Part model, mm, in its own coordinate system. Face numbers are marked on the shaded views. Round coordinates to 2 decimals unless told otherwise and drop trailing zeros. Order: outer loops, then holes, each group sorted by start corner. A loop starts at its lowest first (then second) coordinate and runs counter-clockwise, first axis right, second up. Notation, with made-up numbers: (7, 43) - (23, 43) arc R15 ccw to (23, 71) - close; hole circle Ø7 at (57.5, 6). An arc over 180 degrees is marked (long way). Answer as a JSON object with one key per item and string values.
Autodesk Inventor part; units mm, degrees
ref_plane "Start Plane" through (0, 0, -10) normal (0, 0, 1) x (1, 0, 0)
ref_plane "End Plane" through (0, 0, 140) normal (0, 0, 1) x (1, 0, 0)
ref_plane "Work Plane4" through (0, 0, -10) normal (0, 0, -1) x (-1, 0, 0)
ref_plane "Start Plane" through (0, 0, -10) normal (0, 0, 1) x (1, 0, 0)
ref_plane "End Plane" through (0, 0, 140) normal (0, 0, 1) x (1, 0, 0)
sketch "Sketch" plane through (0, 0, 0) normal (0, 0, 1) x (1, 0, 0)
  line L0 (-10, -7) -> (-10, 7)
  line L1 (-7, 10) -> (7, 10)
  line L2 (10, 7) -> (10, -7)
  line L3 (7, -10) -> (-7, -10)
  arc A0 (-10, -7) -> (-7, -10) centre (-7, -7) ccw
  arc A1 (-7, 10) -> (-10, 7) centre (-7, 7) ccw
  arc A2 (10, 7) -> (7, 10) centre (7, 7) ccw
  arc A3 (7, -10) -> (10, -7) centre (7, -7) ccw
  arc A4 (-7, 8) -> (-8, 7) centre (-7, 7) ccw
  line L4 (-7, 8) -> (7, 8)
  arc A5 (8, 7) -> (7, 8) centre (7, 7) ccw
  line L5 (8, 7) -> (8, -7)
  arc A6 (7, -8) -> (8, -7) centre (7, -7) ccw
  line L6 (7, -8) -> (-7, -8)
  arc A7 (-8, -7) -> (-7, -8) centre (-7, -7) ccw
  line L7 (-8, -7) -> (-8, 7)
  line L8 (0, 14.8698) -> (0, -14.8698) construction
  line L9 (-14.8698, 0) -> (14.8698, 0) construction
  dimension "d7" = 3
  dimension "d10" = 20
  dimension "d11" = 20
  dimension "d12" = 2
  dimension "d15" = 10
  dimension "d16" = 10
extrude "Body" add sketch "Sketch" along normal up to surface (150 mm away) from surface at -10
sketch "Sketch3" plane through (0, 0, 0) normal (0, 0, 1) x (1, 0, 0)
  line L0 (0, 0) -> (10, 0)
ref_plane "Work Plane3" through (0, 0, 0) normal (0, -1, 0) x (1, 0, 0)
sketch "Sketch4" plane through (0, 0, 0) normal (0, -1, 0) x (1, 0, 0)
  line L0 (-2, -10) -> (12, -10)
  line L1 (-2, 140) -> (12, 140)
  dimension "d18" = 150
ref_plane "Work Plane4" through (0, 0, -10) normal (0, 0, -1) x (-1, 0, 0)
split "Split1" plane through (0, 0, -10) removes the side toward (0, 0, -1)
ref_plane "Work Plane5" through (-7, -210, 140) normal (0, 0, 1) x (1, 0, 0)
split "Split2" plane through (-7, -210, 140) removes the side toward (0, 0, 1)
equation "\"d7\" = G_IR"
equation "\"d10\" = G_H"
equation "\"d11\" = G_W"
equation "\"d12\" = G_T"
equation "\"d15\" = 0.5 * d10"
equation "\"d16\" = 0.5 * d11"
equation "\"d3\" = G_L"
equation "\"G_W\" = 20"
equation "\"G_H\" = 20"
equation "\"G_T\" = 2"
equation "\"G_IR\" = 3"
equation "\"G_L\" = d18"
properties part number "ISO 12633-2 - 20x20x2 - 150" material "Steel, Mild"
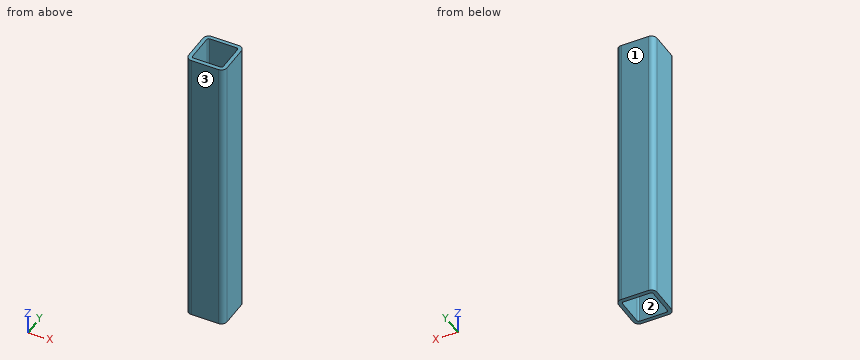
Item 1: Cut at A-A (x = 0.75). Write the cut outline in (y, z).
Taken from the geometry:
{"outline": "(-10, -10) - (-8, -10) - (-8, 140) - (-10, 140) - close; (8, -10) - (10, -10) - (10, 140) - (8, 140) - close"}
Item 2: Two-plate mould, pull along Y, no slides. Class the marked faces 1, 2 and 3: pulls with the +Y half, pulls with the -Y half, needs draft (parallel to the pull), parting line crosses it, or undercut.
Taken from the geometry:
{"face 1": "pulls with the +Y half", "face 2": "undercut", "face 3": "pulls with the -Y half"}
Item 3: Probe L1, parallel to Y at x = 2.5, z = 39; L2, parallel to Y at x = -7.5, z = 66. List the from-to ranges inside material, lowest first. Write a range as from..to.
Taken from the geometry:
{"L1": "-10..-8, 8..10", "L2": "-9.96..-7.87, 7.87..9.96"}
Item 4: Cut at B-B (z = 70.5). Write the cut outline in (x, y).
Taken from the geometry:
{"outline": "(-10, -7) arc R3 ccw to (-7, -10) - (7, -10) arc R3 ccw to (10, -7) - (10, 7) arc R3 ccw to (7, 10) - (-7, 10) arc R3 ccw to (-10, 7) - close; hole (-8, -7) arc R1 ccw to (-7, -8) - (7, -8) arc R1 ccw to (8, -7) - (8, 7) arc R1 ccw to (7, 8) - (-7, 8) arc R1 ccw to (-8, 7) - close"}
